from build123d import *

# Parameters (mm, degrees)
F1_DEPTH  = 1.524
F2_DEPTH  = 19.05
F3_R      = 1.524
F4_R      = 1.524
F5_R      = 1.524
F6_R      = 1.524
F9_DEPTH  = 127
F12_DEPTH = 127
F13_R     = 1.778
F14_DEPTH = 1.524


with BuildPart() as f1:
    # F0 (on Top) → F1 (new body)
    with BuildSketch(Plane.XY):
        Polygon((50.8, 38.1), (38.1, 50.8), (-38.1, 50.8), (-50.8, 38.1), (-50.8, -38.1), (-38.1, -50.8), (38.1, -50.8), (50.8, -38.1), align=None)
        Polygon((-49.276, 35.3134770619), (-49.276, 37.4687385309), (-37.4687385309, 49.276), (-35.3134770619, 49.276), (35.3134770619, 49.276), (37.4687385309, 49.276), (49.276, 37.4687385309), (49.276, 35.3134770619), (49.276, -35.3134770619), (49.276, -37.4687385309), (37.4687385309, -49.276), (35.3134770619, -49.276), (-35.3134770619, -49.276), (-37.4687385309, -49.276), (-49.276, -37.4687385309), (-49.276, -35.3134770619), align=None, mode=Mode.SUBTRACT)
        Polygon((-13.9625229381, 0), (-49.276, 35.3134770619), (-49.276, -35.3134770619), align=None)
        Polygon((-11.8072614691, 0), (-49.276, 37.4687385309), (-49.276, 35.3134770619), (-13.9625229381, 0), (-49.276, -35.3134770619), (-49.276, -37.4687385309), align=None)
        Polygon((-37.4687385309, 49.276), (-49.276, 37.4687385309), (-11.8072614691, 0), (-49.276, -37.4687385309), (-37.4687385309, -49.276), (0, -11.8072614691), (37.4687385309, -49.276), (49.276, -37.4687385309), (11.8072614691, 0), (49.276, 37.4687385309), (37.4687385309, 49.276), (0, 11.8072614691), align=None)
        Polygon((-35.3134770619, 49.276), (-37.4687385309, 49.276), (0, 11.8072614691), (37.4687385309, 49.276), (35.3134770619, 49.276), (0, 13.9625229381), align=None)
        Polygon((49.276, 35.3134770619), (49.276, 37.4687385309), (11.8072614691, 0), (49.276, -37.4687385309), (49.276, -35.3134770619), (13.9625229381, 0), align=None)
        Polygon((35.3134770619, 49.276), (-35.3134770619, 49.276), (0, 13.9625229381), align=None)
        Polygon((0, -11.8072614691), (-37.4687385309, -49.276), (-35.3134770619, -49.276), (0, -13.9625229381), (35.3134770619, -49.276), (37.4687385309, -49.276), align=None)
        Polygon((0, -13.9625229381), (-35.3134770619, -49.276), (35.3134770619, -49.276), align=None)
        Polygon((49.276, -35.3134770619), (49.276, 35.3134770619), (13.9625229381, 0), align=None)
    extrude(amount=-F1_DEPTH)

    # F0 (on Top) → F2 (join)
    with BuildSketch(Plane.XY):
        Polygon((50.8, 38.1), (38.1, 50.8), (-38.1, 50.8), (-50.8, 38.1), (-50.8, -38.1), (-38.1, -50.8), (38.1, -50.8), (50.8, -38.1), align=None)
        Polygon((-49.276, 35.3134770619), (-49.276, 37.4687385309), (-37.4687385309, 49.276), (-35.3134770619, 49.276), (35.3134770619, 49.276), (37.4687385309, 49.276), (49.276, 37.4687385309), (49.276, 35.3134770619), (49.276, -35.3134770619), (49.276, -37.4687385309), (37.4687385309, -49.276), (35.3134770619, -49.276), (-35.3134770619, -49.276), (-37.4687385309, -49.276), (-49.276, -37.4687385309), (-49.276, -35.3134770619), align=None, mode=Mode.SUBTRACT)
        Polygon((-11.8072614691, 0), (-49.276, 37.4687385309), (-49.276, 35.3134770619), (-13.9625229381, 0), (-49.276, -35.3134770619), (-49.276, -37.4687385309), align=None)
        Polygon((-35.3134770619, 49.276), (-37.4687385309, 49.276), (0, 11.8072614691), (37.4687385309, 49.276), (35.3134770619, 49.276), (0, 13.9625229381), align=None)
        Polygon((0, -11.8072614691), (-37.4687385309, -49.276), (-35.3134770619, -49.276), (0, -13.9625229381), (35.3134770619, -49.276), (37.4687385309, -49.276), align=None)
        Polygon((49.276, 35.3134770619), (49.276, 37.4687385309), (11.8072614691, 0), (49.276, -37.4687385309), (49.276, -35.3134770619), (13.9625229381, 0), align=None)
    extrude(amount=F2_DEPTH)

    # F3
    f3_edges = [f1.edges().sort_by_distance(p)[0] for p in [
        (-35.313477, 49.276, 9.525),
        (35.313477, 49.276, 9.525),
        (0, 13.962523, 9.525),
        (0, 11.807261, 9.525),
    ]]
    fillet(f3_edges, radius=F3_R)

    # F4
    f4_edges = [f1.edges().sort_by_distance(p)[0] for p in [
        (-13.962523, 0, 9.525),
        (-11.807261, 0, 9.525),
        (-49.276, 35.313477, 9.525),
        (-49.276, -35.313477, 9.525),
    ]]
    fillet(f4_edges, radius=F4_R)

    # F5
    f5_edges = [f1.edges().sort_by_distance(p)[0] for p in [
        (35.313477, -49.276, 9.525),
        (-35.313477, -49.276, 9.525),
        (0, -13.962523, 9.525),
        (0, -11.807261, 9.525),
    ]]
    fillet(f5_edges, radius=F5_R)

    # F6
    f6_edges = [f1.edges().sort_by_distance(p)[0] for p in [
        (49.276, -35.313477, 9.525),
        (49.276, 35.313477, 9.525),
        (13.962523, 0, 9.525),
        (11.807261, 0, 9.525),
    ]]
    fillet(f6_edges, radius=F6_R)

    # F8 (on offset) → F9 (cut)
    with BuildSketch(Plane(origin=(-44.45, -44.45, 0), x_dir=(0.7071067812, -0.7071067812, 0), z_dir=(-0.7071067812, -0.7071067812, 0))):
        Polygon((-4.3955561211, 8.8357592486), (-4.3955561211, 10.2142407514), (-5.5893561211, 10.9034815027), (-6.7831561211, 10.2142407514), (-6.7831561211, 8.8357592486), (-5.5893561211, 8.1465184973), align=None)
        Polygon((1.7766438789, 8.4984712214), (1.7766438789, 10.5515287786), (-0.0013561211, 11.5780575572), (-1.7793561211, 10.5515287786), (-1.7793561211, 8.4984712214), (-0.0013561211, 7.4719424428), align=None)
        Polygon((-0.0013561211, 11.5780575572), (1.7766438789, 10.5515287786), (1.7766438789, 19.05), (-1.7793561211, 19.05), (-1.7793561211, 10.5515287786), align=None)
        Polygon((6.7804438789, 8.8357592486), (6.7804438789, 10.2142407514), (5.5866438789, 10.9034815027), (4.3928438789, 10.2142407514), (4.3928438789, 8.8357592486), (5.5866438789, 8.1465184973), align=None)
    extrude(amount=-F9_DEPTH, mode=Mode.SUBTRACT)

    # F11 (on offset) → F12 (cut)
    with BuildSketch(Plane(origin=(44.45, -44.45, 0), x_dir=(0.7071067812, 0.7071067812, 0), z_dir=(0.7071067812, -0.7071067812, 0))):
        Polygon((-4.3928438789, 8.8357592486), (-4.3928438789, 10.2142407514), (-5.5866438789, 10.9034815027), (-6.7804438789, 10.2142407514), (-6.7804438789, 8.8357592486), (-5.5866438789, 8.1465184973), align=None)
        Polygon((0.0013561211, 11.5780575572), (1.7793561211, 10.5515287786), (1.7793561211, 19.05), (-1.7766438789, 19.05), (-1.7766438789, 10.5515287786), align=None)
        Polygon((1.7793561211, 8.4984712214), (1.7793561211, 10.5515287786), (0.0013561211, 11.5780575572), (-1.7766438789, 10.5515287786), (-1.7766438789, 8.4984712214), (0.0013561211, 7.4719424428), align=None)
        Polygon((6.7831561211, 8.8357592486), (6.7831561211, 10.2142407514), (5.5893561211, 10.9034815027), (4.3955561211, 10.2142407514), (4.3955561211, 8.8357592486), (5.5893561211, 8.1465184973), align=None)
    extrude(amount=-F12_DEPTH, mode=Mode.SUBTRACT)

    # F13 (on Top) → F14 (cut)
    with BuildSketch(Plane.XY):
        with Locations((-44.45, 0)):
            Circle(F13_R)
        with Locations((0, 44.45)):
            Circle(F13_R)
        with Locations((44.45, 0)):
            Circle(F13_R)
        with Locations((0, -44.45)):
            Circle(F13_R)
    extrude(amount=-F14_DEPTH, mode=Mode.SUBTRACT)


solid = f1.part
The model under review builds one solid part; all positions refer to its coordinate system, in mm. A direction names the side the tool comes from. Give positions to 0.01 mm unless a question says otherwise; leave off trailing zeros. Loops run counter-clockwise (first coordinate to the right, second up) from the corner with the lowest first, then second, coordinate; pieces in that order, holes last. Notation, with made-up numbers: (44.25, 31) -> (82.25, 31) arc R21 ccw to (82.25, 35) -> close; hole circle Ø3 at (-8.75, -20.5). An arc over 180 degrees is marked (long way). Put each result on its own line as item: value. Start each with the question number.
1. Wall thickness on probe 1 along Y at (x, z) = (0, -0.3); probe 2 along Y at (x, z) = (-44.45, -0.8); probe 3 along Y at (x, z) = (-39, 13.75): over which ranges is each line inside the solid? List them lowest first.
2. For faces 1 (the face through (44.54, -43.298, 7.978)), 2 (the face through (-1, -50.8, 9)), list the 3-axis set-ups (+Z, -Z, +X, -X, +Y, -Y) from which the entire face can be reached by the end or side of a thin tool; tool diameter is ignored.
3. Mouldability with a two-part tool opening along Y and no side actions: class faces 3 (the face through (44.5, 44.4, 6.3)), 4 (the face through (31.08, -17.12, 9.39)), 5 (the face through (-50.8, 1, 9)) as released by +Y, released by -Y, zero draft, split by the parting line, or undercut.
4. We need section B-B on y = -24. State the section outline as (x, z) points.
5. Clearance check with flat-ended pins moving along their axes: P1, Ø8, axis at x = 40, y = -28.5, coming from the +Z side; P2, Ø10.5, axis at x = -26.5, y = 0.5, coming from the +Z side. State where each tip first meets the part, or that it passes through.
6. We need section C-C on x = 26.5. State the section outline as (y, z) points, then the cut area to 3 significant figures.
7. We need section A-A on z = 5.5. State how many separate pieces and enclosed holes the cut face has, then the cut area to 3 significant figures.
Determined:
1. probe 1: -50.8 to -46.23, -42.67 to 42.67, 46.23 to 50.8
1. probe 2: -44.45 to -1.78, 1.78 to 44.45
1. probe 3: -49.9 to -47.74, -27.19 to -25.04, 25.04 to 27.19, 47.74 to 49.9
2. face 1: +Z
2. face 2: +Z, -Z, +X, -X, -Y
3. face 3: released by +Y
3. face 4: undercut
3. face 5: zero draft
4. outline: (-50.8, -1.52) -> (50.8, -1.52) -> (50.8, 19.05) -> (49.28, 19.05) -> (49.28, 0) -> (37.96, 0) -> (37.96, 19.05) -> (35.81, 19.05) -> (35.81, 0) -> (12.19, 0) -> (12.19, 19.05) -> (10.04, 19.05) -> (10.04, 0) -> (-10.04, 0) -> (-10.04, 19.05) -> (-12.19, 19.05) -> (-12.19, 0) -> (-35.81, 0) -> (-35.81, 19.05) -> (-37.96, 19.05) -> (-37.96, 0) -> (-49.28, 0) -> (-49.28, 19.05) -> (-50.8, 19.05) -> close
5. P1: z = 19.05
5. P2: z = 0
6. outline: (-50.8, -1.52) -> (50.8, -1.52) -> (50.8, 19.05) -> (49.28, 19.05) -> (49.28, 0) -> (40.46, 0) -> (40.46, 19.05) -> (38.31, 19.05) -> (38.31, 0) -> (14.69, 0) -> (14.69, 19.05) -> (12.54, 19.05) -> (12.54, 0) -> (-12.54, 0) -> (-12.54, 19.05) -> (-14.69, 19.05) -> (-14.69, 0) -> (-38.31, 0) -> (-38.31, 19.05) -> (-40.46, 19.05) -> (-40.46, 0) -> (-49.28, 0) -> (-49.28, 19.05) -> (-50.8, 19.05) -> close
6. area: 377 mm^2
7. separate pieces: 1
7. enclosed holes: 5
7. area: 1,220 mm^2
